Source: three-view drawing plus pictorial views. Frame: mm from the lowest corner of the part. Round coordinates to 2 decimals unless told otherwise and drop trailing zeros. Loops run counter-clockwise (first coordinate to the right, second up) from the corner with the lowest first, then second, coordinate; pieces in that order, holes last. Notation, with made-up numbers: (0, -2) -> (58, -2) arc R14 cw to (58, 2) -> close; hole circle Ø1 at (0.5, -25). An arc over 180 degrees is marked (long way). Answer as a JSON object with one key per item and string values. Group by question number.
Item 1: Material intervals for line 1 (Y direction, x = 12.7, z = 7.75); line 2 (X direction, y = 55.5, z = 10), sorted ascending. Write a range as [from, to].
Item 2: Section query B-B on x = 12.7. Return loops of the section in (y, z).
Item 3: Section query A-A on z = 6.75. Return loops of the section in (x, y).
Item 4: Section query C-C on y = 212.5. Return loops of the section in (x, z).
Item 5: Pin query (flat end, axial travel): pin 1 (3 mm diameter, centred on y = 163, z = 11, fed in from +X); pin 2 (6.5 mm diameter, centred on x = 231, z = 4, fed in from +Y). Return the tip coordinate at first contact, or that it passes through.
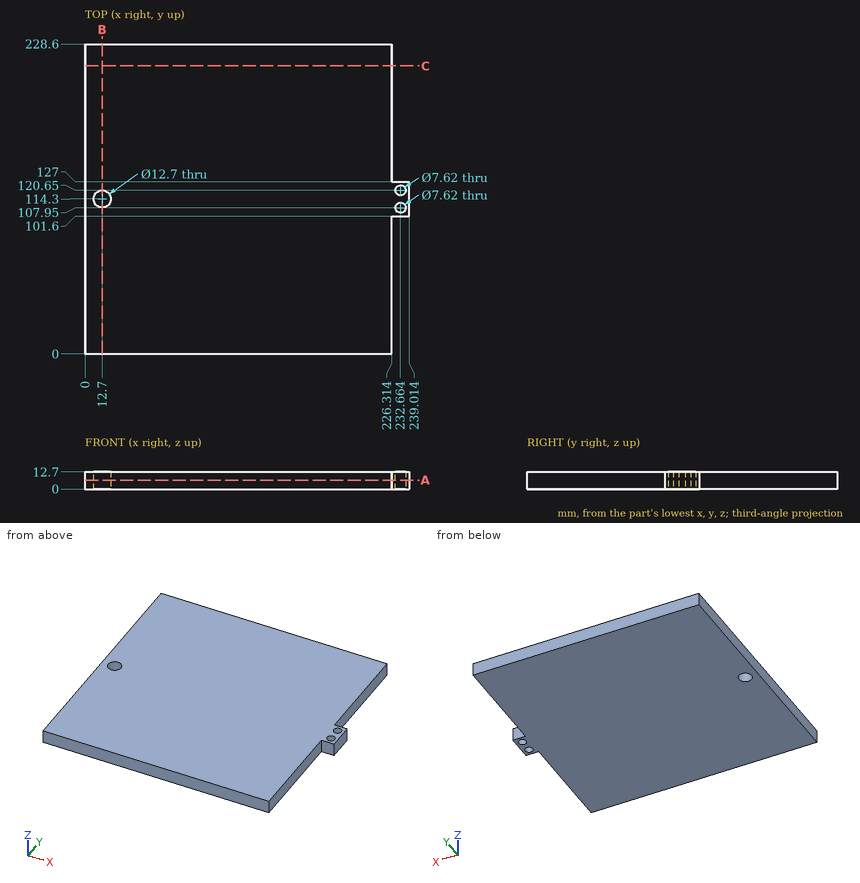
Solved:
{
 "1": {"line 1": "[0, 107.95], [120.65, 228.6]", "line 2": "[0, 226.31]"},
 "2": {"outline": "(0, 0) -> (107.95, 0) -> (107.95, 12.7) -> (0, 12.7) -> close; (120.65, 0) -> (228.6, 0) -> (228.6, 12.7) -> (120.65, 12.7) -> close"},
 "3": {"outline": "(0, 0) -> (226.31, 0) -> (226.31, 101.6) -> (239.01, 101.6) -> (239.01, 127) -> (226.31, 127) -> (226.31, 228.6) -> (0, 228.6) -> close; hole circle Ø12.7 at (12.7, 114.3); hole circle Ø7.62 at (232.66, 107.95); hole circle Ø7.62 at (232.66, 120.65)"},
 "4": {"outline": "(0, 0) -> (226.31, 0) -> (226.31, 12.7) -> (0, 12.7) -> close"},
 "5": {"pin 1": "x = 226.31", "pin 2": "y = 127"}
}
